Could you check a few things on this model? Use its own coordinates, in mm. Face numbers are marked on the shaded views. A direction names the side the tool comes from. Give positions to 0.01 mm unless a question says otherwise; leave off trailing zeros. Order: outer loops, then holes, each group sorted by start corner. A loop starts at its lowest first (then second) coordinate and runs counter-clockwise, first axis right, second up.
(1) Imagine slicing it at D-D, the plane x = 30. Write out the boundary of the cut face in (y, z).
(2) If I drill on probe 1 along X at (y, z) = (-0.5, 5.5); probe 2 along Y at (x, z) = (-31.5, 38.5); probe 3 along Z at (x, y) = (9.5, 5.5), over which ranges is the centre line in solid material (lowest first)?
(3) Imagine slicing it at C-C, the plane y = 28. Write out the boundary of the cut face in (x, z).
(4) If we mould it in two halves opening along Z, with no side actions, what happens to the marked faces 1, 2 and 3? For each: released by +Z, released by -Z, zero draft, split by the parting line, or undercut.
(5) Will these pins go through, and if not, where does the flat tip stop? pin 1 (1.5 mm diameter, centred on x = -27, z = 59, fed in from +Y); pin 2 (0.6 mm diameter, centred on y = 43.5, z = 18.5, fed in from +X); pin 3 (2 mm diameter, centred on x = 30.5, y = -43.5, fed in from +Z).
(6) On a 3-axis mill with a long thin cutter (end or side, diameter ignored), from which of +Z, -Z, +X, -X, +Y, -Y can I reach the whole of each face in a straight line? I mean the marked faces 4 and 5. Say none if no direction works.
(7) Imagine slicing it at A-A, the plane z = 35. Write out the boundary of the cut face in (x, y), then the cut area to 3 significant figures.
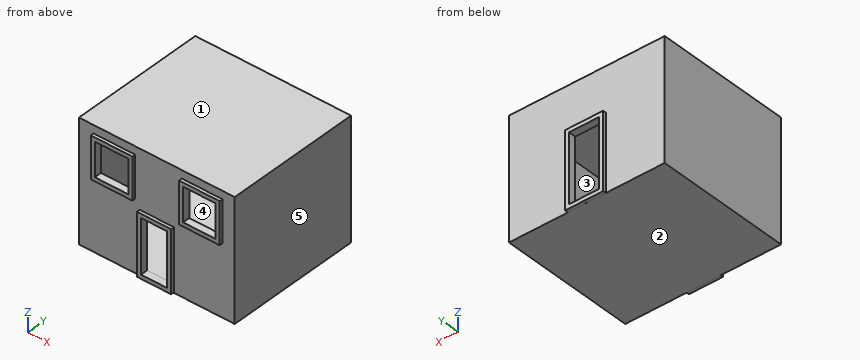
from build123d import *

# Parameters (mm, degrees)
F0_W     = 96.9840660691
F0_H     = 84.8280265927
F1_DEPTH = 75
F2_W     = 21.263839677
F2_H     = 38.4748987854
F3_DEPTH = 2
F4_W     = 25.9946249425
F4_H     = 26.0400751024
F4_W_2   = 25.2393023088
F5_DEPTH = 2
F6_W     = 23.7395130098
F6_H     = 47.4790297449
F7_DEPTH = 2
F8_T     = -2.5


with BuildPart() as f1:
    # F0 (on Top) → F1 (new body)
    with BuildSketch(Plane.XY):
        Rectangle(F0_W, F0_H)
    extrude(amount=F1_DEPTH)

    # F2 (on face) → F3 (join)
    with BuildSketch(Plane.XZ.offset(42.4140132964)):
        with Locations((0, 19.5709709078)):
            Rectangle(F2_W, F2_H)
    extrude(amount=F3_DEPTH)

    # F4 (on face) → F5 (join)
    with BuildSketch(Plane.XZ.offset(42.4140132964)):
        with Locations((-26.4344327152, 56.980330497)):
            Rectangle(F4_W, F4_H)
        with Locations((28.2331126402, 56.980330497)):
            Rectangle(F4_W_2, F4_H)
    extrude(amount=F5_DEPTH)

    # F6 (on face) → F7 (join)
    with BuildSketch(Plane(origin=(0, 42.4140132964, 0), x_dir=(-1, 0, 0), z_dir=(0, 1, 0))):
        with Locations((0, 23.7531457096)):
            Rectangle(F6_W, F6_H)
    extrude(amount=F7_DEPTH)

    # F8
    f8_openings = [f1.faces().sort_by_distance(p)[0] for p in [
        (0, 44.414013, 23.753146),
        (-26.434433, -44.414013, 56.98033),
        (28.233113, -44.414013, 56.98033),
        (0, -44.414013, 19.570971),
    ]]
    offset(amount=F8_T, openings=f8_openings, kind=Kind.INTERSECTION)


solid = f1.part
Answer block:
1. outline: (-44.41, 43.96) - (-42.41, 43.96) - (-42.41, 0) - (42.41, 0) - (42.41, 75) - (-42.41, 75) - (-42.41, 70) - (-44.41, 70) - (-44.41, 67.5) - (-39.91, 67.5) - (-39.91, 72.5) - (39.91, 72.5) - (39.91, 2.5) - (-39.91, 2.5) - (-39.91, 46.46) - (-44.41, 46.46) - close
2. probe 1: x = -48.49 to -45.99, 45.99 to 48.49
2. probe 2: y = -42.41 to -39.91, 39.91 to 42.41
2. probe 3: z = 0 to 2.5, 72.5 to 75
3. outline: (-48.49, 0) - (48.49, 0) - (48.49, 75) - (-48.49, 75) - close; hole (-45.99, 2.5) - (45.99, 2.5) - (45.99, 72.5) - (-45.99, 72.5) - close
4. face 1: released by +Z
4. face 2: released by -Z
4. face 3: undercut
5. pin 1: stops at y = 42.41
5. pin 2: stops at x = 11.87
5. pin 3: stops at z = 70
6. face 4: none
6. face 5: +Z, -Z, +X, +Y, -Y
7. outline: (-48.49, -42.41) - (-10.63, -42.41) - (-10.63, -44.41) - (-8.13, -44.41) - (-8.13, -39.91) - (-45.99, -39.91) - (-45.99, 39.91) - (-9.37, 39.91) - (-9.37, 44.41) - (-11.87, 44.41) - (-11.87, 42.41) - (-48.49, 42.41) - close; (8.13, -44.41) - (10.63, -44.41) - (10.63, -42.41) - (48.49, -42.41) - (48.49, 42.41) - (11.87, 42.41) - (11.87, 44.41) - (9.37, 44.41) - (9.37, 39.91) - (45.99, 39.91) - (45.99, -39.91) - (8.13, -39.91) - close
7. area: 817 mm2
